Geometry check sheet. Reference: the model listing, model coordinates, mm. A direction names the side the tool comes from. Give positions to 0.01 mm unless a question says otherwise; leave off trailing zeros. Loops run counter-clockwise (first coordinate to the right, second up) from the corner with the lowest first, then second, coordinate; pieces in that order, holes last. Notation, with made-up numbers: (76, 33) - (85, 33) arc R31 ccw to (85, 67) - close; hole circle Ø5 at (37.25, 44). An arc over 180 degrees is marked (long way). Use a Markdown table: item, result. Add a question column.
1. Material ranges on L1, parallel to Y at x = 5.75, z = -2.25; L2, parallel to Z at x = -0.25, y = 9.5; L3, parallel to X at y = 45, z = -4.5, recorded low to high.
2. Depth check by flat-ended pin: P1, Ø3, axis at y = 40.5, z = -4, coming from the +X side; P2, Ø3, axis at y = 16, z = -5, coming from the +X side; P3, Ø2, axis at y = 27, z = -1.5, coming from the +X side. Enter the tip coordinate at first touch or a pass-through.
3. Cross-section at C-C on y = 22. Enter the section's corners in (x, z), and give its area (3 significant figures).
4. Set-up check for faces 1 (the cylindrical face through (6.466, 24.164, 2.681)), 2 (the cylindrical face through (-0.54, 49.49, 2.44)): record each of +Z, -Z, +X, -X, +Y, -Y from which the full face is reachable in a straight line by a thin tool's end or side.
5. Cross-section at A-A on z = 0. Enter the section's corners in (x, y).
6. Cross-section at B-B on x = 0. Enter the section's corners in (y, z).
from build123d import *

# Parameters (mm, degrees)
SKETCH1_R           = 7
BOSS_EXTRUDE1_DEPTH = 49
SKETCH2_R           = 2.5
BOSS_EXTRUDE2_DEPTH = 1.5
FILLET1_R           = 0.5


with BuildPart() as part:
    # Sketch1 → Boss-Extrude1 (new body)
    with BuildSketch(Plane(origin=(0, 0, 0), x_dir=(1, 0, 0), z_dir=(0, 1, 0))):
        Circle(SKETCH1_R)
    extrude(amount=BOSS_EXTRUDE1_DEPTH)

    # Sketch2 → Boss-Extrude2 (add)
    with BuildSketch(Plane(origin=(0, 49, 0), x_dir=(1, 0, 0), z_dir=(0, 1, 0))):
        Circle(SKETCH2_R)
    extrude(amount=BOSS_EXTRUDE2_DEPTH)

    # Fillet1
    fillet1_edges = [part.edges().sort_by_distance(p)[0] for p in [
        (-7, 0, 0),
        (-7, 49, 0),
        (-2.5, 50.5, 0),
    ]]
    fillet(fillet1_edges, radius=FILLET1_R)


solid = part.part
Values found:
| question | item | result |
|---|---|---|
| 1 | L1 | y = 0 to 49 |
| 1 | L2 | z = -7 to 7 |
| 1 | L3 | x = -5.36 to 5.36 |
| 2 | P1 | stops at x = 6.54 |
| 2 | P2 | stops at x = 6.06 |
| 2 | P3 | stops at x = 6.98 |
| 3 | outline | circle Ø14 at (0, 0) |
| 3 | area | 154 mm2 |
| 4 | face 1 | +Y, -Y |
| 4 | face 2 | +Y |
| 5 | outline | (-7, 0.5) arc R0.5 ccw to (-6.5, 0) - (6.5, 0) arc R0.5 ccw to (7, 0.5) - (7, 48.5) arc R0.5 ccw to (6.5, 49) - (2.5, 49) - (2.5, 50) arc R0.5 ccw to (2, 50.5) - (-2, 50.5) arc R0.5 ccw to (-2.5, 50) - (-2.5, 49) - (-6.5, 49) arc R0.5 ccw to (-7, 48.5) - close |
| 6 | outline | (0, -6.5) arc R0.5 ccw to (0.5, -7) - (48.5, -7) arc R0.5 ccw to (49, -6.5) - (49, -2.5) - (50, -2.5) arc R0.5 ccw to (50.5, -2) - (50.5, 2) arc R0.5 ccw to (50, 2.5) - (49, 2.5) - (49, 6.5) arc R0.5 ccw to (48.5, 7) - (0.5, 7) arc R0.5 ccw to (0, 6.5) - close |
